Autodesk Inventor part; units mm, degrees
ref_plane "YZ Plane" through (0, 0, 0) normal (1, 0, 0) x (0, 1, 0)
ref_plane "XZ Plane" through (0, 0, 0) normal (0, 1, 0) x (-1, 0, 0)
ref_plane "XY Plane" through (0, 0, 0) normal (0, 0, 1) x (1, 0, 0)
sketch "Sketch1" plane through (0, 0, 0) normal (1, 0, 0) x (0, 1, 0)
  arc A0 (0, -6) -> (0, 6) centre (0, 0) ccw
  line L0 (0, 6) -> (-90, 6)
  line L1 (-90, -6) -> (0, -6)
  arc A1 (-90, 6) -> (-90, -6) centre (-90, 0) ccw
  line L2 (0, 101) -> (0, 6) construction
  line L3 (0, -6) -> (0, -101) construction
  dimension "d1" = 12
  dimension "d3" = 90
extrude "Main Arm" add sketch "Sketch1" along normal blind 10
sketch "Sketch2" plane through (10, 0, 0) normal (1, 0, 0) x (0, 0, -1)
  arc A0 (4.9681, -0.3712) -> (-4.9681, -0.3712) centre (0, 0) ccw
  arc A1 (-3.3596, -21.897) -> (3.3596, -21.897) centre (0, -21.646) ccw
  line L0 (-4.9681, -0.3712) -> (-3.3596, -21.897)
  line L1 (4.9681, -0.3712) -> (3.3596, -21.897)
  point P0 (6, 0)
  dimension "d11" = 9.964
  dimension "d12" = 6.738
  dimension "d13" = 21.646
extrude "Extrusion2" cut sketch "Sketch2" against normal blind 2
sketch "Sketch3" plane through (8, 0, 0) normal (1, 0, 0) x (0, 0, -1)
  circle A0 centre (0, -10.588) radius 0.75
  line L0 (0, 125) -> (0, -125) construction
  circle A1 centre (0, -14.021) radius 0.75
  circle A2 centre (0, -17.454) radius 0.75
  circle A3 centre (0, -20.887) radius 0.75
  point P0 (0, 0)
  dimension "d14" = 1.5
  dimension "d15" = 10.588
  dimension "d19" = 3.433
extrude "Extrusion3" cut sketch "Sketch3" against normal blind 5
sketch "Sketch4" plane through (8, 0, 0) normal (1, 0, 0) x (0, 0, -1)
  circle A0 centre (0, 0) radius 2
  dimension "d26" = 4
extrude "Extrusion4" cut sketch "Sketch4" against normal blind 5.5
sketch "Sketch5" plane through (0, 0, 0) normal (-1, 0, 0) x (0, 0, 1)
  circle A0 centre (0, 0) radius 2
  circle A1 centre (0, 0) radius 2.25
  dimension "d29" = 4.5
extrude "Extrusion5" add sketch "Sketch5" along normal blind 5.5 contours A0
properties part number "Payload Release Actuator Arm"
Design review of the part built by this model. Coordinates are the model's own, in mm. A direction names the side the tool comes from. Give positions to 0.01 mm unless a question says otherwise; leave off trailing zeros. Order: outer loops, then holes, each group sorted by start corner. A loop starts at its lowest first (then second) coordinate and runs counter-clockwise, first axis right, second up.
1. Add section B-B, the plane y = -48. State the section outline as (x, z) points.
Solution:
outline: (0, -6) - (10, -6) - (10, 6) - (0, 6) - close
2. Tool access review of faces 5 (the flat face through (5, -44, 6)), 6 (the flat face through (8, -10, 1)), 7 (the cylindrical face through (-3, 2, 0)): name each direction out of +Z, -Z, +X, -X, +Y, -Y from which nothing blocks a thin tool from reaching the whole face with its end or side.
Solution:
face 5: +Z, +X, -X, +Y, -Y
face 6: +X
face 7: -X
3. For pin 1 Ø4.5 at (y, z) = (0, 0) entering from +X; pin 2 Ø2 at (x, y) = (-1.5, -32) entering from +Z; pin 3 Ø1.7 at (y, z) = (-20.887, 0) entering from -X; pin 4 Ø0.8 at (y, z) = (-21, 0) entering from +X, all flat-tipped, find the tip position at first contact; note any pin that passes through.
Solution:
pin 1: stops at x = 8
pin 2: passes through
pin 3: stops at x = 0
pin 4: stops at x = 3
4. Add section A-A, the plane x = 7. State the section outline as (y, z) points, then the cut area to 3 significant figures.
Solution:
outline: (-90, -6) - (0, -6) arc R6 ccw to (0, 6) - (-90, 6) arc R6 ccw to start; hole circle Ø1.5 at (-20.89, 0); hole circle Ø1.5 at (-17.45, 0); hole circle Ø1.5 at (-14.02, 0); hole circle Ø1.5 at (-10.59, 0); hole circle Ø4 at (0, 0)
area: 1,170 mm2
5. To check wall thickness, follow L1, parallel to Y at x = 5.95, z = 0; L2, parallel to X at y = -14, z = -2.75; L3, parallel to X at y = -53.5, z = -1. State the ranges of each line that lie inside material, in increasing order.
Solution:
L1: y = -96 to -21.64, -20.14 to -18.2, -16.7 to -14.77, -13.27 to -11.34, -9.84 to -2, 2 to 6
L2: x = 0 to 8
L3: x = 0 to 10
6. Mouldability with a two-part tool opening along Z and no side actions: class faces 1 (the flat face through (10, -57, 0)), 2 (the flat face through (2.5, 0, 0)), 3 (the flat face through (9.014, -10.983, -4.175)), 4 (the cylindrical face through (5, 6, 0)) as +Z half, -Z half, draft (parallel to the pull), parting line (faces both ways), or undercut.
Solution:
face 1: draft
face 2: undercut
face 3: undercut
face 4: parting line
